CAD build for the part. Positions are in the model's coordinates, mm. A direction names the side the tool comes from. Round coordinates to 2 decimals unless told otherwise and drop trailing zeros. Write each loop counter-clockwise with the first axis right and the second up, starting at its lowest first coordinate (ties: lowest second). Pieces come first, ordered by that corner, then holes. Notation, with made-up numbers: (10, 85.25) - (58, 85.25) arc R25 ccw to (58, 113.25) - close; hole circle Ø6 at (-22.5, -14.5). An arc over 180 degrees is marked (long way). Use one line per item in the form item = value. Start each with the question number.
Item 1: Drill centre lines: L1, parallel to Y at x = 48, z = 0.2; L2, parallel to Y at x = 30.5, z = 0.3; L3, parallel to X at y = 122.5, z = 0.3. Where is each one in solid material? Low to high.
Item 2: Band-saw the part on D-D, the plane y = 72.5. List the corners of the cut face in (x, z), and give its area (3 significant figures).
Item 3: Band-saw the part on C-C, the plane x = -27. List the corners of the cut face in (y, z), and give its area (3 significant figures).
Item 4: Pull direction X, two halves, no side cores. Call faces 1 (the flat face through (-2, 2, 0)), 2 (the flat face through (-104.28, -39.42, 0.25)), 3 (the cylindrical face through (-19.527, 148.724, 0.246)): +X half, -X half, draft (parallel to the pull), parting line (faces both ways), or undercut.
Item 5: Tool access for faces 4 (the flat face through (-2, 2, 0.5)), 5 (the flat face through (-100.776, -16.908, 0.254)): list every direction of +Z, -Z, +X, -X, +Y, -Y with a clear straight run to the whole face (end or side of a thin tool).
Item 6: Band-saw the part on B-B, the plane z = 0.2. Give the number of separate pieces and of enclosed holes in the cut face, and give its area (3 significant figures).
Item 7: Band-saw the part on A-A, the plane x = 39. List the corners of the cut face in (y, z).
from build123d import *

# Parameters (mm, degrees)
ESQUISSE1_R             = 150
BOSS_EXTRU_1_DEPTH      = 0.5
ESQUISSE6_W             = 35
ESQUISSE6_H             = 29
ENL_V_MAT_EXTRU_2_DEPTH = 3.175
ESQUISSE7_R             = 2.1
ENL_V_MAT_EXTRU_3_DEPTH = 213.132623611


with BuildPart() as part:
    # Esquisse1 → Boss.-Extru.1 (new body)
    with BuildSketch(Plane.XY):
        Circle(ESQUISSE1_R)
    extrude(amount=BOSS_EXTRU_1_DEPTH)

    # Esquisse6 → Enlèv. mat.-Extru.2 (cut)
    with BuildSketch(Plane.XY.offset(0.5)):
        with Locations((35.5, 110.228215567)):
            Rectangle(ESQUISSE6_W, ESQUISSE6_H)
        Polygon((73.90306654, -63.452565052), (56.40306654, -93.763454184), (81.51780325, -108.263454184), (99.01780325, -77.952565052), align=None)
        Polygon((-109.40306654, -1.964761383), (-91.90306654, -32.275650515), (-117.01780325, -46.775650515), (-134.51780325, -16.464761383), align=None)
    extrude(amount=-ENL_V_MAT_EXTRU_2_DEPTH, mode=Mode.SUBTRACT)

    # Esquisse7 → Enlèv. mat.-Extru.3 (cut, through all)
    with BuildSketch(Plane.XY.offset(0.5)):
        with Locations((-133.660108095, -41.950332968)):
            Circle(ESQUISSE7_R)
        with Locations((-87.760761694, -15.450332968)):
            Circle(ESQUISSE7_R)
        with Locations((30.5, 136.728215567)):
            Circle(ESQUISSE7_R)
        with Locations((30.5, 83.728215567)):
            Circle(ESQUISSE7_R)
        with Locations((103.160108095, -94.777882599)):
            Circle(ESQUISSE7_R)
        with Locations((57.260761694, -68.277882599)):
            Circle(ESQUISSE7_R)
    extrude(amount=-ENL_V_MAT_EXTRU_3_DEPTH, mode=Mode.SUBTRACT)


solid = part.part
Determined:
q1.L1 = -142.11 to 95.73, 124.73 to 142.11
q1.L2 = -146.87 to 81.63, 85.83 to 95.73, 124.73 to 134.63, 138.83 to 146.87
q1.L3 = -86.57 to 18, 53 to 86.57
q2.outline = (-131.32, 0) - (131.32, 0) - (131.32, 0.5) - (-131.32, 0.5) - close
q2.area = 131 mm²
q3.outline = (-147.55, 0) - (147.55, 0) - (147.55, 0.5) - (-147.55, 0.5) - close
q3.area = 148 mm²
q4.face_1 = draft
q4.face_2 = undercut
q4.face_3 = parting line
q5.face_4 = +Z, +X, -X, +Y, -Y
q5.face_5 = +Z, -Z
q6.separate_pieces = 1
q6.enclosed_holes = 9
q6.area = 67,600 mm²
q7.outline = (-144.84, 0) - (95.73, 0) - (95.73, 0.5) - (-144.84, 0.5) - close; (124.73, 0) - (144.84, 0) - (144.84, 0.5) - (124.73, 0.5) - close
